Part model, mm, in its own coordinate system. Face numbers are marked on the shaded views. A direction names the side the tool comes from. Coordinates: 2 decimals unless noted, no trailing zeros. Loops run counter-clockwise (first coordinate to the right, second up) from the corner with the lowest first, then second, coordinate; pieces in that order, holes last. Notation, with made-up numbers: M -5.75,0.25 L 24.25,0.25 A17 ccw 24.25,12.25 Z; hole C 89,-14.5 d9. An arc over 180 degrees is marked long. Use CSV: the item, a comma, the result in double quotes. Start each with the question number.
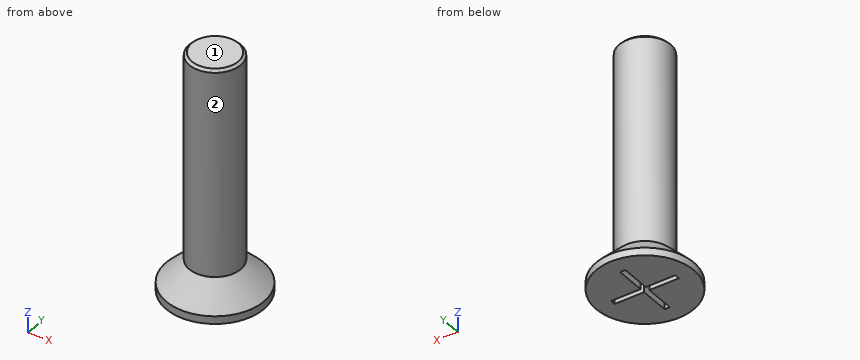
from build123d import *

# Parameters (mm, degrees)
BOX_W             = 0.2
BOX_H             = 2.5
BOX_DEPTH         = 0.5
BOX001_W          = 2.5
BOX001_H          = 0.2
BOX001_DEPTH      = 0.5
CYLINDER_R        = 1.9
CYLINDER_DEPTH    = 1.2
CYLINDER001_R     = 1
CYLINDER001_DEPTH = 9.2
CHAMFER_SIZE      = 0.8999
CHAMFER001_SIZE   = 0.1


with BuildPart() as obj1:
    # Box → Box (new body)
    with BuildSketch(Plane(origin=(-0.1, -1.25, 0), x_dir=(1, 0, 0), z_dir=(0, 0, 1))):
        with Locations((0.1, 1.25)):
            Rectangle(BOX_W, BOX_H)
    extrude(amount=BOX_DEPTH)


with BuildPart() as fusion:
    # Box001 → Box001 (new body)
    with BuildSketch(Plane(origin=(-1.25, -0.1, 0), x_dir=(1, 0, 0), z_dir=(0, 0, 1))):
        with Locations((1.25, 0.1)):
            Rectangle(BOX001_W, BOX001_H)
    extrude(amount=BOX001_DEPTH)

    # Fusion: union obj1
    add(obj1.part)


with BuildPart() as zylinder:
    # Cylinder → Cylinder (new body)
    with BuildSketch(Plane.XY):
        Circle(CYLINDER_R)
    extrude(amount=CYLINDER_DEPTH)


with BuildPart() as screw:
    # Cylinder001 → Cylinder001 (new body)
    with BuildSketch(Plane.XY.offset(0.1)):
        Circle(CYLINDER001_R)
    extrude(amount=CYLINDER001_DEPTH)

    # Fusion001: union Zylinder
    add(zylinder.part)

    # Cut: cut Fusion
    add(fusion.part, mode=Mode.SUBTRACT)

    # Chamfer
    chamfer_edges = [screw.edges().sort_by_distance(p)[0] for p in [
        (-1.9, 0, 1.2),
    ]]
    chamfer(chamfer_edges, length=CHAMFER_SIZE)

    # Chamfer001
    chamfer001_edges = [screw.edges().sort_by_distance(p)[0] for p in [
        (-1, 0, 9.3),
    ]]
    chamfer(chamfer001_edges, length=CHAMFER001_SIZE)


solid = screw.part
1. Tool access for the marked faces 1 and 2: list every direction of +Z, -Z, +X, -X, +Y, -Y with a clear straight run to the whole face (end or side of a thin tool).
2. Wall check: probe 1 along X at (y, z) = (-1.05, 0.75); probe 2 along Z at (x, y) = (-0.4, 0). Give the ranges that are in metal, low to high.
3. Slice it at C-C, the plane z = 1.5. List the corners of the cut face in (x, y).
4. Pin check, flat tips, straight feed: pin 1 (1.5 mm diameter, centred on x = 1.5, z = 1.5, fed in from +Y); pin 2 (2 mm diameter, centred on y = -0.5, z = 3.5, fed in from +X); pin 3 (0.6 mm diameter, centred on y = -0.5, z = 0, fed in from -X). Stop position of each tip, or through.
Found:
1,face 1,"+Z, +X, -X, +Y, -Y"
1,face 2,"+Z"
2,probe 1,"-1 to 1"
2,probe 2,"0.5 to 9.3"
3,outline,"C 0,0 d2"
4,pin 1,"y = 0.77"
4,pin 2,"x = 1"
4,pin 3,"x = -1.89"
